The listing builds one solid part. Answer for the finished solid, in the listing's coordinates (mm). A direction names the side the tool comes from. Round coordinates to 2 decimals unless told otherwise and drop trailing zeros. Order: outer loops, then holes, each group sorted by start corner. A loop starts at its lowest first (then second) coordinate and runs counter-clockwise, first axis right, second up. Notation, with made-up numbers: (28, 11) -> (77, 11) arc R13 cw to (77, 29) -> close; hole circle Ø2 at (57.5, -11). An arc over 180 degrees is marked (long way). Answer in a Markdown table with one row per item. Add a question column.
```python
from build123d import *

# Parameters (mm, degrees)
BOSS_EXTRUDE5_DEPTH = 23
SKETCH3_W           = 3.5
SKETCH3_H           = 1
BOSS_EXTRUDE7_DEPTH = 42.2
CUT_EXTRUDE3_DEPTH  = 42.2
CUT_EXTRUDE4_DEPTH  = 42.2
FILLET1_R           = 3
FILLET2_R           = 3
FILLET3_R           = 0.5
FILLET4_R           = 0.5
FILLET5_R           = 3
FILLET6_R           = 3
CUT_EXTRUDE5_DEPTH  = 42.2
CUT_EXTRUDE6_DEPTH  = 42.2
CUT_EXTRUDE7_DEPTH  = 42.2


with BuildPart() as part:
    # Sketch1 → Boss-Extrude5 (new body)
    with BuildSketch(Plane(origin=(0, 0, 0), x_dir=(1, 0, 0), z_dir=(0, 1, 0))):
        Polygon((-53, 0), (53, 0), (53, 3), (24.1, 3), (24.1, 45.2), (21.1, 45.2), (21.1, 3), (-21.1, 3), (-21.1, 45.2), (-24.1, 45.2), (-24.1, 3), (-53, 3), align=None)
    extrude(amount=BOSS_EXTRUDE5_DEPTH)

    # Sketch3 → Boss-Extrude7 (add)
    with BuildSketch(Plane(origin=(0, 0, -3), x_dir=(-1, 0, 0), z_dir=(0, 0, -1))):
        with Locations((-19.35, 22.5)):
            Rectangle(SKETCH3_W, SKETCH3_H)
        with Locations((19.35, 22.5)):
            Rectangle(SKETCH3_W, SKETCH3_H)
    extrude(amount=BOSS_EXTRUDE7_DEPTH)

    # Sketch5 → Cut-Extrude3 (cut)
    with BuildSketch(Plane(origin=(0, 22, 0), x_dir=(-1, 0, 0), z_dir=(0, -1, 0))):
        with BuildLine():
            Line((-18.35, 43.490720045), (-18.35, 4.709279955))
            ThreePointArc((-18.35, 4.709279955), (-19.35, 3.709279955), (-20.35, 4.709279955))
            Line((-20.35, 4.709279955), (-20.35, 43.490720045))
            ThreePointArc((-20.35, 43.490720045), (-19.35, 44.490720045), (-18.35, 43.490720045))
        make_face()
    extrude(amount=-CUT_EXTRUDE3_DEPTH, mode=Mode.SUBTRACT)

    # Sketch5<4> → Cut-Extrude4 (cut)
    with BuildSketch(Plane(origin=(0, 22, 0), x_dir=(-1, 0, 0), z_dir=(0, -1, 0))):
        with BuildLine():
            Line((18.35, 4.709279955), (18.35, 43.490720045))
            ThreePointArc((18.35, 43.490720045), (19.35, 44.490720045), (20.35, 43.490720045))
            Line((20.35, 43.490720045), (20.35, 4.709279955))
            ThreePointArc((20.35, 4.709279955), (19.35, 3.709279955), (18.35, 4.709279955))
        make_face()
    extrude(amount=-CUT_EXTRUDE4_DEPTH, mode=Mode.SUBTRACT)

    # Fillet1
    fillet1_edges = [part.edges().sort_by_distance(p)[0] for p in [
        (-24.1, 11.5, -45.2),
    ]]
    fillet(fillet1_edges, radius=FILLET1_R)

    # Fillet2
    fillet2_edges = [part.edges().sort_by_distance(p)[0] for p in [
        (24.1, 11.5, -45.2),
    ]]
    fillet(fillet2_edges, radius=FILLET2_R)

    # Fillet3
    fillet3_edges = [part.edges().sort_by_distance(p)[0] for p in [
        (-17.6, 22.5, -45.2),
    ]]
    fillet(fillet3_edges, radius=FILLET3_R)

    # Fillet4
    fillet4_edges = [part.edges().sort_by_distance(p)[0] for p in [
        (17.6, 22.5, -45.2),
    ]]
    fillet(fillet4_edges, radius=FILLET4_R)

    # Fillet5
    fillet5_edges = [part.edges().sort_by_distance(p)[0] for p in [
        (53, 11.5, -3),
    ]]
    fillet(fillet5_edges, radius=FILLET5_R - 0.0001)  # a hair under: the kernel refuses the full size

    # Fillet6
    fillet6_edges = [part.edges().sort_by_distance(p)[0] for p in [
        (-53, 11.5, -3),
    ]]
    fillet(fillet6_edges, radius=FILLET6_R - 0.0001)  # a hair under: the kernel refuses the full size

    # Sketch6 → Cut-Extrude5 (cut)
    with BuildSketch(Plane(origin=(0, 0, -3), x_dir=(-1, 0, 0), z_dir=(0, 0, -1))):
        with BuildLine():
            Line((-27.05, 15.25), (-47.05, 15.25))
            ThreePointArc((-47.05, 15.25), (-49.05, 17.25), (-47.05, 19.25))
            Line((-47.05, 19.25), (-27.05, 19.25))
            ThreePointArc((-27.05, 19.25), (-25.05, 17.25), (-27.05, 15.25))
        make_face()
        with BuildLine():
            Line((-27.05, 3.75), (-47.05, 3.75))
            ThreePointArc((-47.05, 3.75), (-49.05, 5.75), (-47.05, 7.75))
            Line((-47.05, 7.75), (-27.05, 7.75))
            ThreePointArc((-27.05, 7.75), (-25.05, 5.75), (-27.05, 3.75))
        make_face()
    extrude(amount=-CUT_EXTRUDE5_DEPTH, mode=Mode.SUBTRACT)

    # Sketch7 → Cut-Extrude6 (cut)
    with BuildSketch(Plane(origin=(0, 0, -3), x_dir=(-1, 0, 0), z_dir=(0, 0, -1))):
        with BuildLine():
            Line((47.05, 15.25), (27.05, 15.25))
            ThreePointArc((27.05, 15.25), (25.05, 17.25), (27.05, 19.25))
            Line((27.05, 19.25), (47.05, 19.25))
            ThreePointArc((47.05, 19.25), (49.05, 17.25), (47.05, 15.25))
        make_face()
    extrude(amount=-CUT_EXTRUDE6_DEPTH, mode=Mode.SUBTRACT)

    # Sketch7<3> → Cut-Extrude7 (cut)
    with BuildSketch(Plane(origin=(0, 0, -3), x_dir=(-1, 0, 0), z_dir=(0, 0, -1))):
        with BuildLine():
            Line((27.05, 7.503040911), (47.05, 7.503040911))
            ThreePointArc((47.05, 7.503040911), (49.05, 5.503040911), (47.05, 3.503040911))
            Line((47.05, 3.503040911), (27.05, 3.503040911))
            ThreePointArc((27.05, 3.503040911), (25.05, 5.503040911), (27.05, 7.503040911))
        make_face()
    extrude(amount=-CUT_EXTRUDE7_DEPTH, mode=Mode.SUBTRACT)


solid = part.part
```
Item 1: A tool of negligible diameter and unlimited length cuts with its end or side. For faces 4 (the face through (49.05, 5.71, -1.52)), 5 (the face through (21.1, 11, -24)), 6 (the face through (23.2, 11.66, -44.34)), from which of +Z, -Z, +X, -X, +Y, -Y can it reach the whole face along a straight path? Write none if from no direction.
Item 2: The part is cut by section C-C, the plane y = 17.25. State how many separate pieces and enclosed holes the cut face has, and give its area (3 significant figures).
Item 3: For a pull along Y with two mould halves and no side action, classify faces 1 (the face through (-18, 22, -24)), 2 (the face through (-25.05, 5.46, -1.52)), 3 (the face through (-1, 11, 0)) as released by +Y, released by -Y, zero draft, split by the parting line, or undercut.
Item 4: The part is cut by section B-B, the plane z = -39.5. Give the vertices of the cut face in (x, y).
Item 5: Flat-ended cylindrical pins translate along their axes: P1, Ø6.5, axis at y = 14, z = -18.5, coming from the +X side; P2, Ø12, axis at y = 9, z = -8.5, coming from the -X side; P3, Ø11.5, axis at x = -3.5, y = 11.5, coming from the -Z side. Find the tip coordinate at first contact, or state that the pin passes through.
Item 6: The part is cut by section A-A, the plane x = -19.35. Give the vertices of the cut face in (y, z), and give its area (3 significant figures).
Item 7: Find the intervals of material crossed by probe 1 along X at (y, z) = (5, -34); probe 2 along X at (y, z) = (22.25, -42.5); probe 3 along Z at (x, y) = (-34.5, 10.5), in increasing order. Write a range as [from, to].
Resolved:
| question | item | result |
|---|---|---|
| 1 | face 4 | +Z, -Z |
| 1 | face 5 | -Z, -Y |
| 1 | face 6 | -Z, +X, +Y, -Y |
| 2 | separate pieces | 3 |
| 2 | enclosed holes | 0 |
| 2 | area | 419 mm2 |
| 3 | face 1 | released by -Y |
| 3 | face 2 | undercut |
| 3 | face 3 | zero draft |
| 4 | outline | (-24.1, 0) -> (-21.1, 0) -> (-21.1, 22) -> (-20.35, 22) -> (-20.35, 23) -> (-24.1, 23) -> close; (-18.35, 22) -> (-17.6, 22) -> (-17.6, 23) -> (-18.35, 23) -> close; (17.6, 22) -> (18.35, 22) -> (18.35, 23) -> (17.6, 23) -> close; (20.35, 22) -> (21.1, 22) -> (21.1, 0) -> (24.1, 0) -> (24.1, 23) -> (20.35, 23) -> close |
| 5 | P1 | x = 24.1 |
| 5 | P2 | x = -51.66 |
| 5 | P3 | z = -3 |
| 6 | outline | (0, -3) -> (22, -3) -> (22, -3.71) -> (23, -3.71) -> (23, 0) -> (0, 0) -> close; (22, -45.2) -> (23, -45.2) -> (23, -44.49) -> (22, -44.49) -> close |
| 6 | area | 70.4 mm2 |
| 7 | probe 1 | [-24.1, -21.1], [21.1, 24.1] |
| 7 | probe 2 | [-24.08, -20.35], [-18.35, -17.6], [17.6, 18.35], [20.35, 24.08] |
| 7 | probe 3 | [-3, 0] |
